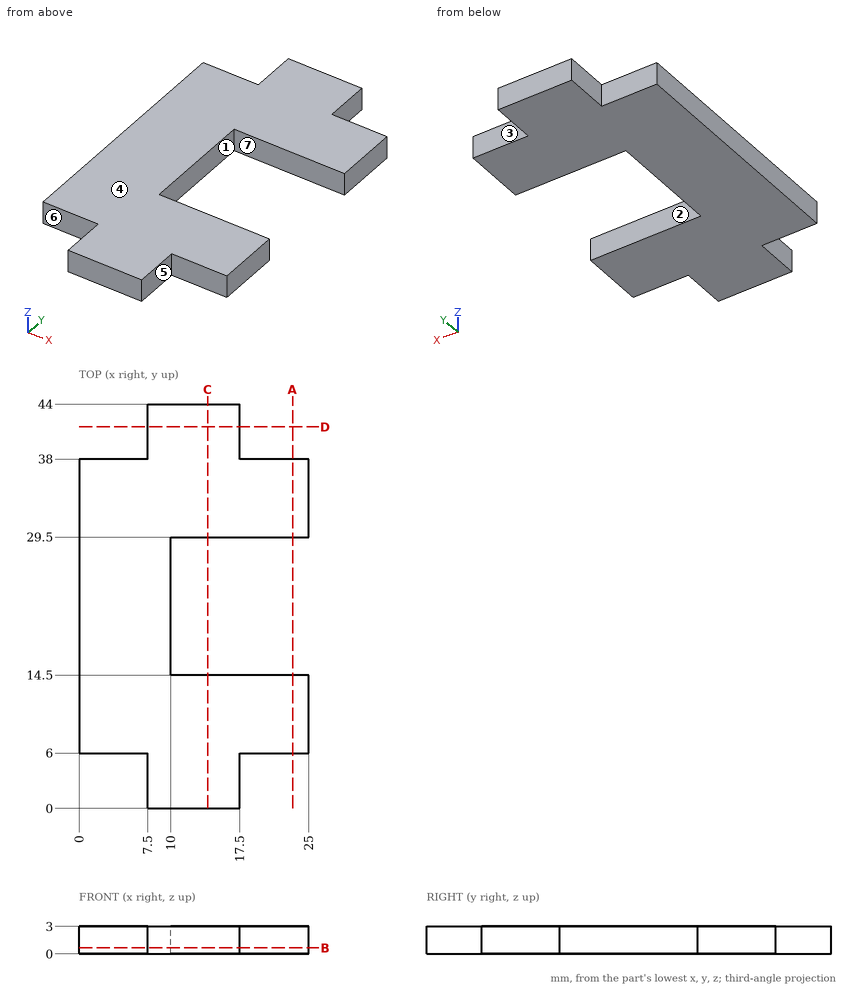
Check sheet for the drawn part. Datum: minimum x, y, z corner. Units: mm. A direction names the side the tool comes from. Coordinates: 2 decimals unless noted, no trailing zeros. Order: outer loops, then holes, each group sorted by start corner. A loop starts at its lowest first (then second) coordinate and runs counter-clockwise, first axis right, second up. Notation, with made-up numbers: M 15.5,-27 L 39.5,-27 A10 ccw 39.5,-23 Z; hole C -14.5,-27.75 d10. An arc over 180 degrees is marked long. One line per item, written item: value. Start each with the question number.
Item 1: Sectioned sample at C-C (x = 14). Enter the section's corners in (y, z).
Item 2: Sectioned sample at B-B (z = 0.65). Enter the section's corners in (x, y).
Item 3: Scan lines: probe 1 along Y at (x, z) = (13, 2.5); probe 2 along Y at (x, z) = (22.75, 2.4); probe 3 along Y at (x, z) = (3.25, 2.15). Record each from-to range of solid material in increasing order.
Item 4: Access from +Z, -Z, +X, -X, +Y, -Y to the whole of each face (thin tool, end or side, straight path). Record for the marked faces 5, 6 and 7.
Item 5: Gauge pin test, flat ends, axial feed: pin 1 (1.5 mm diameter, centred on y = 4.5, z = 1, fed in from +X); pin 2 (0.9 mm diameter, centred on x = 22, z = 2, fed in from -Y); pin 3 (0.9 mm diameter, centred on y = 2.5, z = 2, fed in from -X). Record the tip position at first contact, or that the pin passes through.
Item 6: Mould release check, pull along Y, two halves, no side actions. Record for the marked faces 1, 2, 3 and 4: released by +Y, released by -Y, zero draft, split by the parting line, or undercut.
Item 7: Sectioned sample at D-D (y = 41.5). Enter the section's corners in (x, z), then the cut area to 3 significant figures.
Item 8: Sectioned sample at A-A (x = 23.25). Enter the section's corners in (y, z), then the cut area to 3 significant figures.
Conclusion:
1. outline: M 0,0 L 14.5,0 L 14.5,3 L 0,3 Z; M 29.5,0 L 44,0 L 44,3 L 29.5,3 Z
2. outline: M 0,6 L 7.5,6 L 7.5,0 L 17.5,0 L 17.5,6 L 25,6 L 25,14.5 L 10,14.5 L 10,29.5 L 25,29.5 L 25,38 L 17.5,38 L 17.5,44 L 7.5,44 L 7.5,38 L 0,38 Z
3. probe 1: y = 0 to 14.5, 29.5 to 44
3. probe 2: y = 6 to 14.5, 29.5 to 38
3. probe 3: y = 6 to 38
4. face 5: +Z, -Z, +X, -Y
4. face 6: +Z, -Z, -X, -Y
4. face 7: +Z, -Z, +X
5. pin 1: stops at x = 17.5
5. pin 2: stops at y = 6
5. pin 3: stops at x = 7.5
6. face 1: undercut
6. face 2: undercut
6. face 3: released by +Y
6. face 4: zero draft
7. outline: M 7.5,0 L 17.5,0 L 17.5,3 L 7.5,3 Z
7. area: 30.0 mm^2
8. outline: M 6,0 L 14.5,0 L 14.5,3 L 6,3 Z; M 29.5,0 L 38,0 L 38,3 L 29.5,3 Z
8. area: 51.0 mm^2
